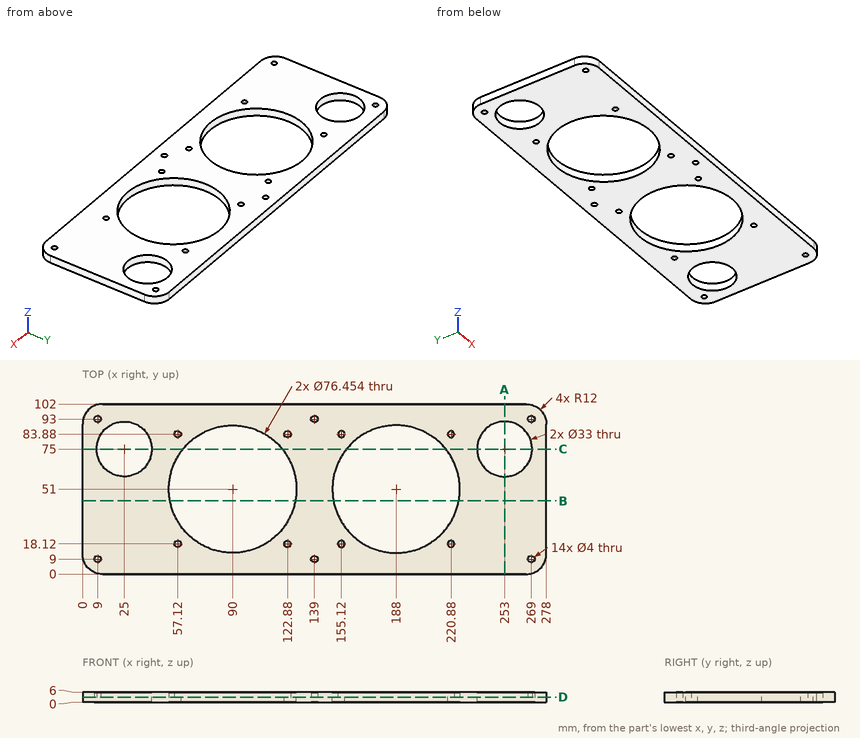
Check sheet for the drawn part. Datum: minimum x, y, z corner. Units: mm. Round coordinates to 2 decimals unless told otherwise and drop trailing zeros. Order: outer loops, then holes, each group sorted by start corner. A loop starts at its lowest first (then second) coordinate and runs counter-clockwise, first axis right, second up. Notation, with made-up numbers: (-29.5, 30) - (20.5, 30) arc R23 cw to (20.5, 51) - close; hole circle Ø2 at (57.25, 1.25). An arc over 180 degrees is marked (long way). Use a Markdown table: item, result. Add a question column.
(1) Sectioned sample at C-C, the plane y = 75. Enter the section's corners in (x, z).
(2) Sectioned sample at D-D, the plane z = 3. Count the separate pieces of the cut face and the enclosed holes in it, and give its area (3 significant figures).
(3) Sectioned sample at A-A, the plane x = 253. Enter the section's corners in (y, z).
(4) Sectioned sample at B-B, the plane y = 44. Enter the section's corners in (x, z).
(5) Material ranges on line 1 along X through (y, z) = (47, 4.25); line 2 along X through (y, z) = (86, 3.4) (1 decimal); line 3 along X through (y, z) = (45, 1), recorded low to high. Write a range as [from, to].
Answers below:
| question | item | result |
|---|---|---|
| 1 | outline | (0, 0) - (8.5, 0) - (8.5, 6) - (0, 6) - close; (41.5, 0) - (60.25, 0) - (60.25, 6) - (41.5, 6) - close; (119.75, 0) - (158.25, 0) - (158.25, 6) - (119.75, 6) - close; (217.75, 0) - (236.5, 0) - (236.5, 6) - (217.75, 6) - close; (269.5, 0) - (278, 0) - (278, 6) - (269.5, 6) - close |
| 2 | separate pieces | 1 |
| 2 | enclosed holes | 18 |
| 2 | area | 17,200 mm² |
| 3 | outline | (0, 0) - (58.5, 0) - (58.5, 6) - (0, 6) - close; (91.5, 0) - (102, 0) - (102, 6) - (91.5, 6) - close |
| 4 | outline | (0, 0) - (52.42, 0) - (52.42, 6) - (0, 6) - close; (127.58, 0) - (150.42, 0) - (150.42, 6) - (127.58, 6) - close; (225.58, 0) - (278, 0) - (278, 6) - (225.58, 6) - close |
| 5 | line 1 | [0, 51.98], [128.02, 149.98], [226.02, 278] |
| 5 | line 2 | [0, 12.7], [37.3, 74.6], [105.4, 172.6], [203.4, 240.7], [265.3, 278] |
| 5 | line 3 | [0, 52.25], [127.75, 150.25], [225.75, 278] |
